from build123d import *

# Parameters (mm, degrees)
F0_R     = 2
F1_DEPTH = 65
F2_R     = 2
F2_R_2   = 1.5
F3_DEPTH = 10
F4_R     = 2
F4_R_2   = 1.5
F5_DEPTH = 10


with BuildPart() as f1:
    # F0 (on Front) → F1 (new body, symmetric)
    with BuildSketch(Plane.XZ):
        Circle(F0_R)
    extrude(amount=F1_DEPTH, both=True)

    # F2 (on face) → F3 (cut)
    with BuildSketch(Plane.XZ.offset(65)):
        Circle(F2_R)
        Circle(F2_R_2, mode=Mode.SUBTRACT)
    extrude(amount=-F3_DEPTH, mode=Mode.SUBTRACT)

    # F4 (on face) → F5 (cut)
    with BuildSketch(Plane(origin=(0, 65, 0), x_dir=(-1, 0, 0), z_dir=(0, 1, 0))):
        Circle(F4_R)
        Circle(F4_R_2, mode=Mode.SUBTRACT)
    extrude(amount=-F5_DEPTH, mode=Mode.SUBTRACT)


solid = f1.part
Here's how the part is built. I have some questions about the finished solid (model axes, mm). A direction names the side the tool comes from. Give positions to 0.01 mm unless a question says otherwise; leave off trailing zeros. Write each loop counter-clockwise with the first axis right and the second up, starting at its lowest first coordinate (ties: lowest second). Pieces come first, ordered by that corner, then holes. Notation, with made-up numbers: (36, -22.5) -> (46, -22.5) arc R17 ccw to (46, 6.5) -> close; hole circle Ø6 at (74.25, 52.5). An arc over 180 degrees is marked (long way). Use one line per item in the form item = value. Start each with the question number.
1. If I drill on L1, parallel to Z at x = 1.35, y = -21; L2, parallel to Y at x = -0.75, z = 1.55; L3, parallel to X at y = 31, z = 1.3, over which ranges is the centre line in solid material (lowest first)?
2. Imagine slicing it at B-B on z = 0. List the corners of the cut face in (x, y) for me, plus the area to 3 significant figures.
3. Imagine slicing it at C-C on y = -9. List the corners of the cut face in (x, z) for me.
4. On a 3-axis mill with a long thin cutter (end or side, diameter ignored), from which of +Z, -Z, +X, -X, +Y, -Y can I reach the whole of each face in a straight line? I mean faces 1 (the face through (0, -1, -2)), 2 (the face through (-1.5, -60.07, 0.07)), 3 (the face through (1.5, 60.07, 0.07)). Say none if no direction works.
5. Imagine slicing it at A-A on x = 0. List the corners of the cut face in (y, z) for me.
Entries:
q1.L1 = -1.48 to 1.48
q1.L2 = -55 to 55
q1.L3 = -1.52 to 1.52
q2.outline = (-2, -55) -> (-1.5, -55) -> (-1.5, -65) -> (1.5, -65) -> (1.5, -55) -> (2, -55) -> (2, 55) -> (1.5, 55) -> (1.5, 65) -> (-1.5, 65) -> (-1.5, 55) -> (-2, 55) -> close
q2.area = 500 mm²
q3.outline = circle Ø4 at (0, 0)
q4.face_1 = +Y, -Y
q4.face_2 = -Y
q4.face_3 = +Y
q5.outline = (-65, -1.5) -> (-55, -1.5) -> (-55, -2) -> (55, -2) -> (55, -1.5) -> (65, -1.5) -> (65, 1.5) -> (55, 1.5) -> (55, 2) -> (-55, 2) -> (-55, 1.5) -> (-65, 1.5) -> close
